Input: part model. Units: mm. Frame: model coordinates. A direction names the side the tool comes from. Give positions to 0.01 mm unless a question says otherwise; leave off trailing zeros. Loops run counter-clockwise (first coordinate to the right, second up) from the corner with the lowest first, then second, coordinate; pieces in that order, holes last. Notation, with made-up numbers: (6.25, 45.25) - (15.25, 45.25) arc R27 cw to (15.25, 74.25) - close; hole circle Ø2 at (65, -38). An arc over 180 degrees is marked (long way). Answer as a JSON object with one key per item and string values.
from build123d import *

# Parameters (mm, degrees)
F0_W     = 10
F0_H     = 32
F1_DEPTH = 5
F3_DEPTH = 10.001


with BuildPart() as f1:
    # F0 (on Top) → F1 (new body)
    with BuildSketch(Plane.XY):
        Rectangle(F0_W, F0_H)
    extrude(amount=F1_DEPTH)

    # F2 (on face) → F3 (cut, through all)
    with BuildSketch(Plane.YZ.offset(5)):
        Polygon((-12.05, 1), (-12.05, 0), (12.05, 0), (12.05, 1), (14.05, 1), (14.05, 3.05), (-14.05, 3.05), (-14.05, 1), align=None)
    extrude(amount=-F3_DEPTH, mode=Mode.SUBTRACT)


solid = f1.part
Item 1: Cut plane A-A (z = 0.7). Return loops of the section in (x, y), then the cut area to 3 significant figures.
Geometry check:
{"outline": "(-5, -16) - (5, -16) - (5, -12.05) - (-5, -12.05) - close; (-5, 12.05) - (5, 12.05) - (5, 16) - (-5, 16) - close", "area": "79.0 mm2"}
Item 2: Material intervals for line 1 (Y direction, x = 0, z = 1.5); line 2 (Y direction, x = -3.75, z = 0.2); line 3 (Z direction, x = -4.5, y = -7), sorted ascending. Write a range as [from, to].
Geometry check:
{"line 1": "y = [-16, -14.05], [14.05, 16]", "line 2": "y = [-16, -12.05], [12.05, 16]", "line 3": "z = [3.05, 5]"}
Item 3: Cut plane B-B (y = 13). Return loops of the section in (x, z), then the cut area to 3 significant figures.
Geometry check:
{"outline": "(-5, 0) - (5, 0) - (5, 1) - (-5, 1) - close; (-5, 3.05) - (5, 3.05) - (5, 5) - (-5, 5) - close", "area": "29.5 mm2"}
Item 4: Contact query for a flat-ended pin moving along its axis: P1, Ø5, axis at x = 1, y = -5, coming from the -Z side. Output: stop coordinate, or through.
Geometry check:
{"P1": "stops at z = 3.05"}
Item 5: Cut plane C-C (x = -2.75). Return loops of the section in (y, z), then the cut area to 3 significant figures.
Geometry check:
{"outline": "(-16, 0) - (-12.05, 0) - (-12.05, 1) - (-14.05, 1) - (-14.05, 3.05) - (14.05, 3.05) - (14.05, 1) - (12.05, 1) - (12.05, 0) - (16, 0) - (16, 5) - (-16, 5) - close", "area": "78.3 mm2"}
Item 6: Cut plane D-D (y = 1.5). Return loops of the section in (x, z).
Geometry check:
{"outline": "(-5, 3.05) - (5, 3.05) - (5, 5) - (-5, 5) - close"}
Item 7: Mould query, pull axis Z, two halves, no side actions, for faces 1 (the face through (0, 14.05, 2)), 2 (the face through (0, 0, 5)), 3 (the face through (0, -14, 0)). Classes: released by +Z, released by -Z, zero draft, split by the parting line, or undercut.
Geometry check:
{"face 1": "undercut", "face 2": "released by +Z", "face 3": "released by -Z"}
Item 8: Access query for faces 4 (the face through (0.1, -12.05, 0.5)), 5 (the face through (0, 16, 2)), 6 (the face through (0, 13, 1)). Directions: +Z, -Z, +X, -X, +Y, -Y. A direction counts if a zero-diameter tool reaches every point of the face in a straight line with its end or side. Return the directions, or none.
Geometry check:
{"face 4": "-Z, +X, -X", "face 5": "+Z, -Z, +X, -X, +Y", "face 6": "+X, -X"}
